from build123d import *

# Parameters (mm, degrees)
BOSS_EXTRUDE1_START     = -109.223144111
BOSS_EXTRUDE1_OUTLINE_R = 6.35
BOSS_EXTRUDE1_DEPTH     = 109.223144111


# Read off the part's stored shape, not the designer's step: Boss-Extrude1
with BuildPart() as part:
    # Boss-Extrude1 outline → Boss-Extrude1 (new body)
    with BuildSketch(Plane.XY.offset(89.157144111).offset(BOSS_EXTRUDE1_START)):
        Circle(BOSS_EXTRUDE1_OUTLINE_R)
    extrude(amount=BOSS_EXTRUDE1_DEPTH)


solid = part.part
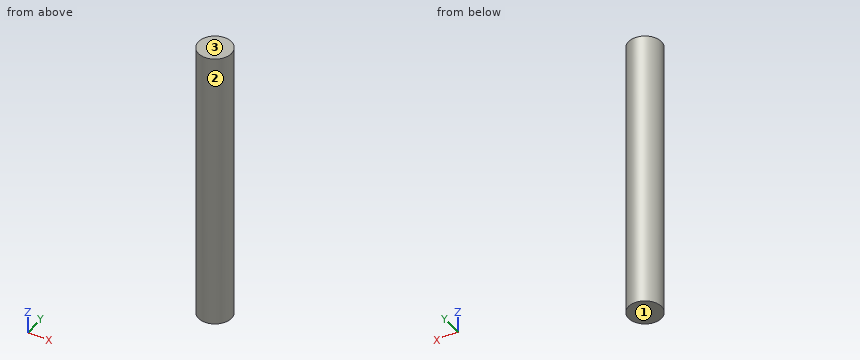
The model under review builds one solid part; all positions refer to its coordinate system, in mm. Face numbers are marked on the shaded views. Round coordinates to 2 decimals unless told otherwise and drop trailing zeros. Order: outer loops, then holes, each group sorted by start corner. A loop starts at its lowest first (then second) coordinate and runs counter-clockwise, first axis right, second up. Notation, with made-up numbers: (45.5, 7) -> (50.5, 7) arc R19 cw to (50.5, 22) -> close; hole circle Ø6 at (-37.5, 81.25). An arc over 180 degrees is marked (long way). Return JSON: item names as keys, results as strings.
1. Take a section at A-A (z = -3.5). Write out the cut boundary in (x, y), then the cut area to 3 significant figures.
Answer block:
{"outline": "circle Ø12.7 at (0, 0)", "area": "127 mm²"}
2. For L1, parallel to X at y = 0.25, z = -4; L2, parallel to Y at x = 0.5, z = 63; L3, parallel to Y at x = 4.5, z = 11.5, list the stretches that pass through material, from the lowest coordinate up. Write a range as [from, to].
Answer block:
{"L1": "x = [-6.35, 6.35]", "L2": "y = [-6.33, 6.33]", "L3": "y = [-4.48, 4.48]"}
3. The part is to be moulded in two halves that separate along Z. For the marked faces 1, 2 and 3, say which applies: +Z half, -Z half, draft (parallel to the pull), parting line (faces both ways), or undercut.
Answer block:
{"face 1": "-Z half", "face 2": "draft", "face 3": "+Z half"}
4. Take a section at C-C (x = 4.5). Write out the cut boundary in (y, z).
Answer block:
{"outline": "(-4.48, -20.07) -> (4.48, -20.07) -> (4.48, 89.16) -> (-4.48, 89.16) -> close"}
5. Take a section at B-B (y = -1.5). Write out the cut boundary in (x, z).
Answer block:
{"outline": "(-6.17, -20.07) -> (6.17, -20.07) -> (6.17, 89.16) -> (-6.17, 89.16) -> close"}
6. Insertion check: P1, Ø3, axis at x = 2.5, z = -5.5, coming from the +Y side; P2, Ø2, axis at x = 4, z = 59, coming from the -Y side; P3, Ø1, axis at x = 2, z = 31.5, coming from the +Y side; P4, Ø1, axis at x = -0.5, z = 28.5, coming from the -Y side. Each pin has a flat end and moves straight along its axis. Give the tip position at first contact, or say it passes through.
Answer block:
{"P1": "stops at y = 6.27", "P2": "stops at y = -5.6", "P3": "stops at y = 6.17", "P4": "stops at y = -6.35"}
